Work out the finished part from the listing and answer in its coordinate system (mm). A direction names the side the tool comes from. Give positions to 0.01 mm unless a question says otherwise; leave off trailing zeros. Order: outer loops, then holes, each group sorted by start corner. A loop starts at its lowest first (then second) coordinate and runs counter-clockwise, first axis right, second up.
```python
from build123d import *

# Parameters (mm, degrees)
SKETCH1_W           = 111.125
SKETCH1_H           = 53.975
BOSS_EXTRUDE1_DEPTH = 32.54375
SKETCH2_W           = 27.78125
SKETCH2_H           = 19.05
CUT_EXTRUDE1_DEPTH  = 3.175
SKETCH4_R           = 5.55625
BOSS_EXTRUDE2_DEPTH = 23.8125
SKETCH5_R           = 1.7859375
BOSS_EXTRUDE3_DEPTH = 3.175


with BuildPart() as part:
    # Sketch1 → Boss-Extrude1 (new body)
    with BuildSketch(Plane(origin=(0, 0, 0), x_dir=(1, 0, 0), z_dir=(0, 1, 0))):
        with Locations((55.5625, 26.9875)):
            Rectangle(SKETCH1_W, SKETCH1_H)
    extrude(amount=BOSS_EXTRUDE1_DEPTH)

    # Sketch2 → Cut-Extrude1 (cut)
    with BuildSketch(Plane.ZY):
        with Locations((-32.146875, 15.875)):
            Rectangle(SKETCH2_W, SKETCH2_H)
    extrude(amount=-CUT_EXTRUDE1_DEPTH, mode=Mode.SUBTRACT)

    # Sketch4 → Boss-Extrude2 (add)
    with BuildSketch(Plane(origin=(111.125, 0, 0), x_dir=(0, 0, -1), z_dir=(1, 0, 0))):
        with Locations((9.525, 16.271875)):
            Circle(SKETCH4_R)
    extrude(amount=BOSS_EXTRUDE2_DEPTH)

    # Sketch5 → Boss-Extrude3 (add)
    with BuildSketch(Plane(origin=(134.9375, 0, 0), x_dir=(0, 0, -1), z_dir=(1, 0, 0))):
        with Locations((9.525, 16.271875)):
            Circle(SKETCH5_R)
    extrude(amount=BOSS_EXTRUDE3_DEPTH)


solid = part.part
```
1. Given P1, Ø1.5, axis at y = 6, z = -33, coming from the +X side (3 decimals); P2, Ø9.5, axis at y = 17.5, z = -29, coming from the -X side (3 decimals), each flat-ended and moving along its own axis, determine where each tip first touches the part or whether it passes through.
Findings below:
P1: stops at x = 111.125
P2: stops at x = 3.175
2. Straight lines are drawn through the part: probe 1 along X at (y, z) = (6, -51) (3 decimals); probe 2 along X at (y, z) = (18.5, -40.5) (3 decimals). For each, find the intervals that lie inside material, in ascending order.
Findings below:
probe 1: x = 0 to 111.125
probe 2: x = 3.175 to 111.125
3. The part is cut by section A-A (y = 24). Write down the section's boundary in (x, z) (1 decimal).
Findings below:
outline: (0, -54) - (111.1, -54) - (111.1, 0) - (0, 0) - (0, -18.3) - (3.2, -18.3) - (3.2, -46) - (0, -46) - close
4. The part is cut by section D-D (x = 123.5). Write down the section's boundary in (y, z) (1 decimal), then the cut area to 3 significant figures.
Findings below:
outline: circle Ø11.1 at (16.3, -9.5)
area: 97.0 mm2
5. The part is cut by section B-B (z = -42). Write down the section's boundary in (x, y) (3 decimals), then the cut area to 3 significant figures.
Findings below:
outline: (0, 0) - (111.125, 0) - (111.125, 32.544) - (0, 32.544) - (0, 25.4) - (3.175, 25.4) - (3.175, 6.35) - (0, 6.35) - close
area: 3,560 mm2
6. The mould has two halves that part along Y. Classify faces 1 (the face through (55, 0, -27)), 2 (the face through (134.938, 18, -8)), 3 (the face through (2, 16, -18.256)): pulls with the +Y half, pulls with the -Y half, needs draft (parallel to the pull), parting line crosses it, or undercut.
Findings below:
face 1: pulls with the -Y half
face 2: needs draft
face 3: undercut
7. Which of the six approach directions +Z, -Z, +X, -X, +Y, -Y give full straight-line access (tool end or side, diameter ignored) to faces 4 (the face through (55, 16, -53.975)), 5 (the face through (136.503, 18.043, -9.293)), 6 (the face through (2, 25.4, -32))?
Findings below:
face 4: -Z, +X, -X, +Y, -Y
face 5: +X
face 6: -X
8. The part is cut by section C-C (z = -17). Write down the section's boundary in (x, y) (3 decimals).
Findings below:
outline: (0, 0) - (111.125, 0) - (111.125, 32.544) - (0, 32.544) - close
